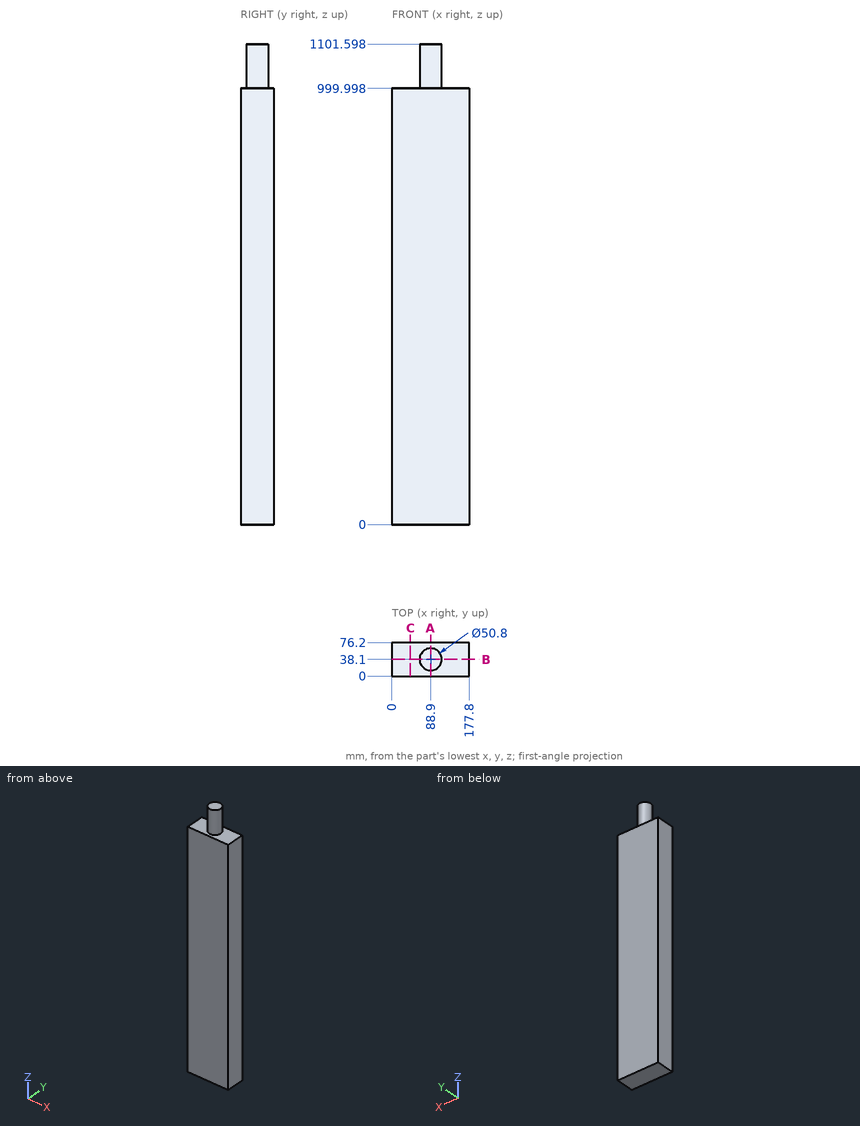
Print and shaded views of the part. All mm, measured from the part's lowest x, y and z. Coordinates: 2 decimals unless noted, no trailing zeros. Write each loop counter-clockwise with the first axis right and the second up, starting at its lowest first coordinate (ties: lowest second). Pieces come first, ordered by that corner, then holes.
(1) Cut at B-B, the plane y = 38.1. List the corners of the cut face in (x, z), and give its area (3 significant figures).
(2) Cut at C-C, the plane x = 42.5. List the corners of the cut face in (y, z).
(3) Cut at A-A, the plane x = 88.9. List the corners of the cut face in (y, z).
(4) Flat gauge pins, fed straight in: pin 1 (3 mm diameter, centred on y = 53, z = 383, fed in from -X); pin 2 (5 mm diameter, centred on x = 56.5, y = 53.5, fed in from +Z). Where does each tip first touch, or does it go through?
(5) Drill centre line: probe 1 along Z at (x, y) = (106, 14). Where is it in solid material? Low to high.
Geometry says:
1. outline: (0, 0) - (177.8, 0) - (177.8, 1000) - (114.3, 1000) - (114.3, 1101.6) - (63.5, 1101.6) - (63.5, 1000) - (0, 1000) - close
1. area: 183,000 mm2
2. outline: (0, 0) - (76.2, 0) - (76.2, 1000) - (0, 1000) - close
3. outline: (0, 0) - (76.2, 0) - (76.2, 1000) - (63.5, 1000) - (63.5, 1101.6) - (12.7, 1101.6) - (12.7, 1000) - (0, 1000) - close
4. pin 1: stops at x = 0
4. pin 2: stops at z = 1000
5. probe 1: z = 0 to 1000
